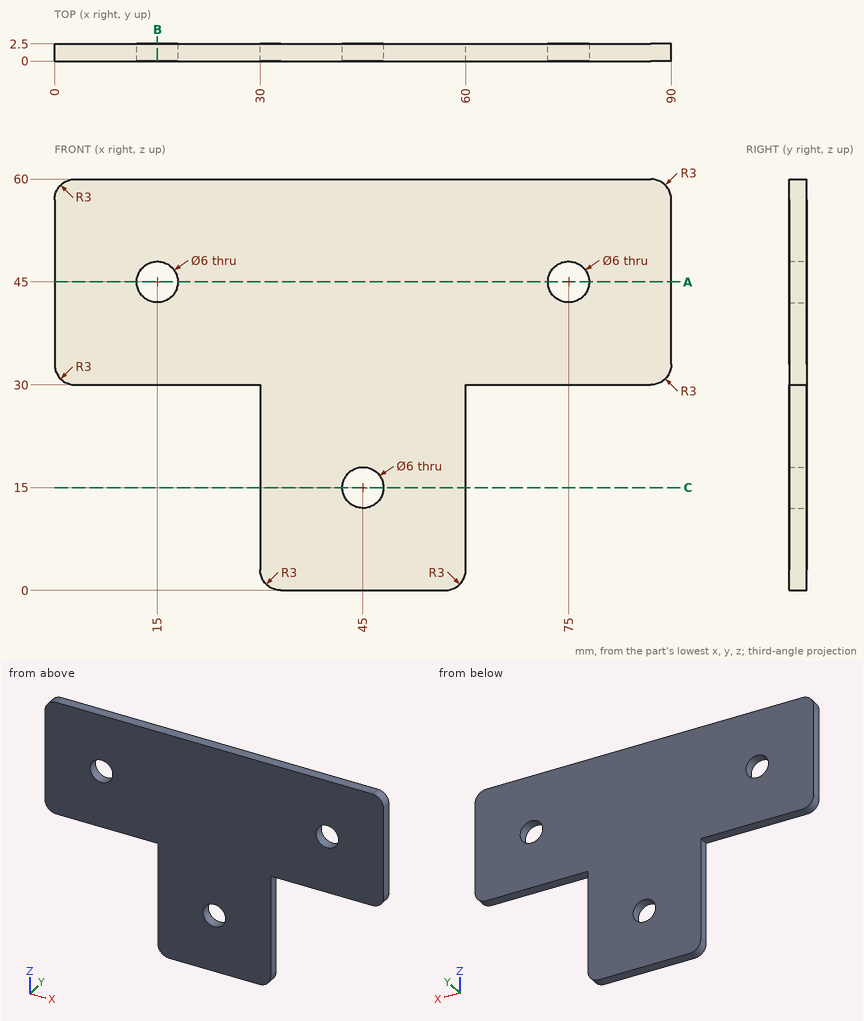
Geometry check sheet. Reference: drawing and pictorial views, mm from the part's lowest x, y, z. Give positions to 0.01 mm unless a question says otherwise; leave off trailing zeros. Write each loop counter-clockwise with the first axis right and the second up, starting at its lowest first coordinate (ties: lowest second). Pieces come first, ordered by that corner, then holes. Notation, with made-up numbers: (36, -26) - (61, -26) arc R23 ccw to (61, -7) - close; hole circle Ø3 at (-13, 66.25). An arc over 180 degrees is marked (long way). Put each result on its own line as item: value.
Q1. Depth check by flat-ended pin: P1, Ø1.5, axis at x = 16, y = 0.5, coming from the -Z side; P2, Ø6, axis at x = 43.5, z = 25.5, coming from the -Y side; P3, Ø1, axis at y = 2, z = 28.5, coming from the +X side. Enter the tip coordinate at first touch or a pass-through.
Result:
P1: z = 30
P2: y = 0
P3: x = 60
Q2. Scan lines: probe 1 along Z at (x, y) = (45, 1.5); probe 2 along X at (y, z) = (2.25, 47.5); probe 3 along Z at (x, y) = (5, 0.2). Record each from-to range of solid material in increasing order. Write a range as from..to.
Result:
probe 1: 0..12, 18..60
probe 2: 0..13.34, 16.66..73.34, 76.66..90
probe 3: 30..60
Q3. Section check B-B on x = 15. Record the cut outline in (y, z).
Result:
outline: (0, 30) - (2.5, 30) - (2.5, 42) - (0, 42) - close; (0, 48) - (2.5, 48) - (2.5, 60) - (0, 60) - close
Q4. Section check A-A on z = 45. Record the cut outline in (x, y).
Result:
outline: (0, 0) - (12, 0) - (12, 2.5) - (0, 2.5) - close; (18, 0) - (72, 0) - (72, 2.5) - (18, 2.5) - close; (78, 0) - (90, 0) - (90, 2.5) - (78, 2.5) - close
Q5. Section check C-C on z = 15. Record the cut outline in (x, y).
Result:
outline: (30, 0) - (42, 0) - (42, 2.5) - (30, 2.5) - close; (48, 0) - (60, 0) - (60, 2.5) - (48, 2.5) - close
